Geometry: see drawing. Coordinates: mm, zero at the bounding-box minimum. Coordinates: 2 decimals unless noted, no trailing zeros. Write each loop counter-clockwise with the first axis right and the second up, starting at its lowest first coordinate (ties: lowest second). Pieces come first, ordered by that corner, then holes.
1) Section query C-C (x = 40.5). Output: boundary loops of the cut face in (y, z), then the cut area to 3 significant figures.
2) Line query: L1, parallel to X at y = 78, z = 2.5 (1 decimal); L2, parallel to X at y = 78.5, z = 2.2 (1 decimal); L3, parallel to X at y = 47.5, z = 2.7 (1 decimal). Output: solid intervals per line, ascending.
3) Section query B-B (z = 1.05). Output: boundary loops of the cut face in (x, y) (1 decimal).
4) Pin query (flat end, axial travel): pin 1 Ø1.5 at (x, z) = (40, 1.5) entering from +Y; pin 2 Ø3 at (x, y) = (14.62, 98.66) entering from -Z. Return the tip coordinate at first contact, or that it passes through.
5) Section query D-D (x = 107). Output: boundary loops of the cut face in (y, z).
6) Section query A-A (x = 15). Output: boundary loops of the cut face in (y, z), then the cut area to 3 significant figures.
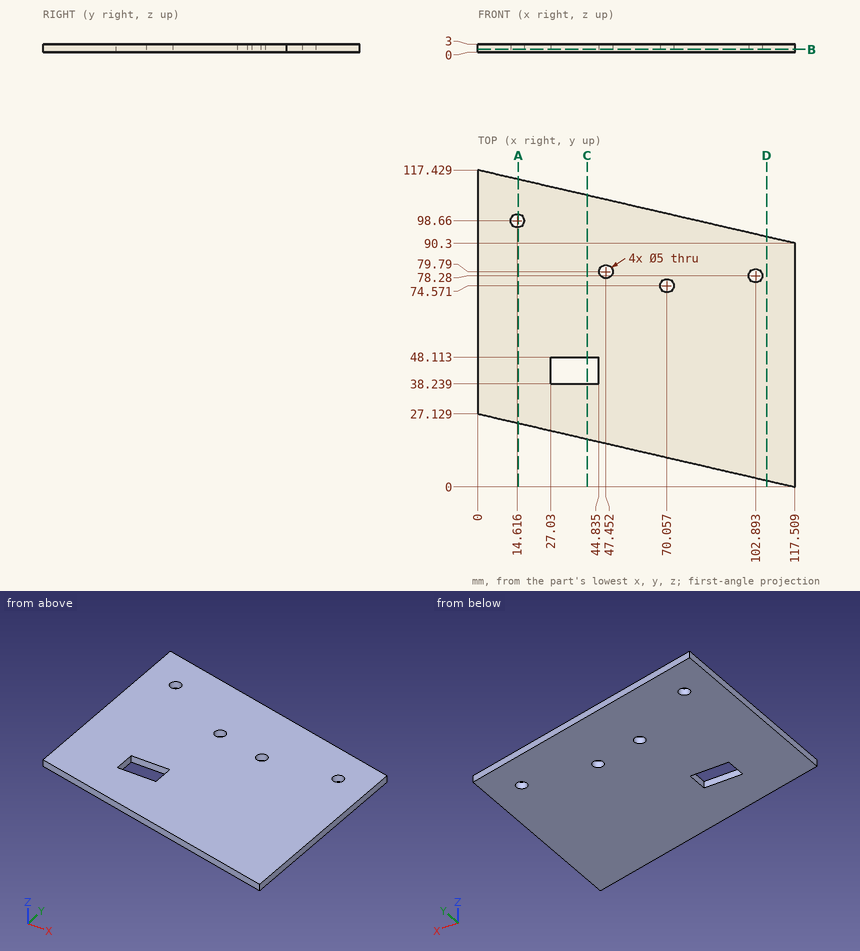
Answer:
1. outline: (17.78, 0) - (38.24, 0) - (38.24, 3) - (17.78, 3) - close; (48.11, 0) - (108.08, 0) - (108.08, 3) - (48.11, 3) - close
1. area: 241 mm2
2. L1: x = 0 to 45.7, 49.2 to 100.4, 105.4 to 117.5
2. L2: x = 0 to 45.3, 49.6 to 100.4, 105.4 to 117.5
2. L3: x = 0 to 27, 44.8 to 117.5
3. outline: (0, 27.1) - (117.5, 0) - (117.5, 90.3) - (0, 117.4) - close; hole circle Ø5 at (14.6, 98.7); hole (27, 38.2) - (44.8, 38.2) - (44.8, 48.1) - (27, 48.1) - close; hole circle Ø5 at (47.5, 79.8); hole circle Ø5 at (70.1, 74.6); hole circle Ø5 at (102.9, 78.3)
4. pin 1: stops at y = 108.37
4. pin 2: passes through
5. outline: (2.43, 0) - (92.73, 0) - (92.73, 3) - (2.43, 3) - close
6. outline: (23.67, 0) - (96.19, 0) - (96.19, 3) - (23.67, 3) - close; (101.13, 0) - (113.97, 0) - (113.97, 3) - (101.13, 3) - close
6. area: 256 mm2
